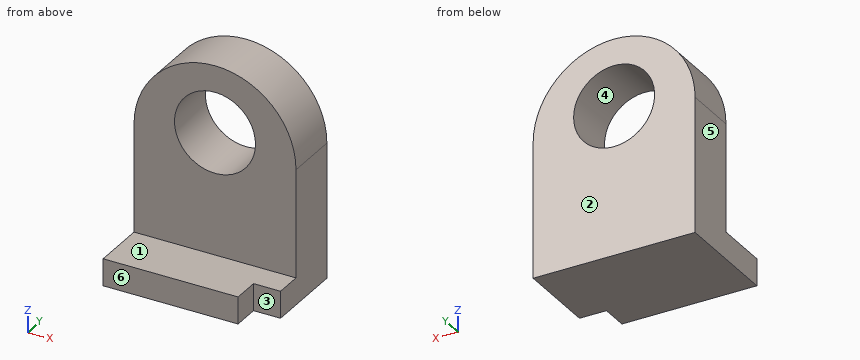
from build123d import *

# Parameters (mm, degrees)
F0_W     = 76.2
F0_H     = 50.8
F1_DEPTH = 12.7
F2_W     = 12.7
F2_H     = 12.7
F3_DEPTH = 12.7
F5_DEPTH = 25.4
F6_R     = 19.05
F7_DEPTH = 25.4


with BuildPart() as f1:
    # F0 (on Top) → F1 (new body)
    with BuildSketch(Plane.XY):
        Rectangle(F0_W, F0_H)
    extrude(amount=F1_DEPTH)

    # F2 (on face) → F3 (cut)
    with BuildSketch(Plane.XY.offset(12.7)):
        with Locations((31.75, -19.05)):
            Rectangle(F2_W, F2_H)
    extrude(amount=-F3_DEPTH, mode=Mode.SUBTRACT)

    # F4 (on Front) → F5 (join)
    with BuildSketch(Plane.XZ):
        with BuildLine():
            Line((-38.1, 12.7), (38.1, 12.7))
            Line((38.1, 12.7), (38.1, 63.5))
            ThreePointArc((38.1, 63.5), (0, 25.4), (-38.1, 63.5))
            Line((-38.1, 63.5), (-38.1, 12.7))
        make_face()
        with BuildLine():
            ThreePointArc((-38.1, 63.5), (0, 25.4), (38.1, 63.5))
            Line((38.1, 63.5), (-38.1, 63.5))
        make_face()
        with BuildLine():
            Line((-38.1, 63.5), (38.1, 63.5))
            ThreePointArc((38.1, 63.5), (0, 101.6), (-38.1, 63.5))
        make_face()
    extrude(amount=-F5_DEPTH)

    # F6 (on face) → F7 (cut)
    with BuildSketch(Plane.XZ):
        with Locations((0, 70.110589)):
            Circle(F6_R)
    extrude(amount=-F7_DEPTH, mode=Mode.SUBTRACT)


solid = f1.part
Can you work these out from the model? Positions are in its coordinate system, mm. Face numbers are marked on the shaded views. A direction names the side the tool comes from. Round coordinates to 2 decimals unless told otherwise and drop trailing zeros. Loops run counter-clockwise (first coordinate to the right, second up) from the corner with the lowest first, then second, coordinate; pieces in that order, holes last. Notation, with made-up numbers: (59, 53.25) - (94, 53.25) arc R14 cw to (94, 71.25) - close; hole circle Ø7 at (63.5, -34.5). An arc over 180 degrees is marked (long way). Write item = value, one per line. Start each with the question number.
(1) If we mould it in two halves opening along X, with no side actions, what happens to the marked faces 4, 5 and 6? For each: released by +X, released by -X, zero draft, split by the parting line, or undercut.
(2) If I drill on probe 1 along Z at (x, y) = (0, 18.75); probe 2 along Y at (x, z) = (5.5, 43.5); probe 3 along Z at (x, y) = (-6, 13), over which ranges is the centre line in solid material (lowest first)? Write a range as [from, to].
(3) For the marked faces 1, 2 and 3, which set-ups out of +Z, -Z, +X, -X, +Y, -Y let a thin tool reach every point of the face, with its end or its side?
(4) For P1, Ø7.5, axis at x = -1, y = -17, coming from the +Z side; P2, Ø14, axis at x = 33, z = 9, coming from the -Y side; P3, Ø3, axis at x = -3.5, z = 45, coming from the -Y side; P4, Ø12, axis at y = -2.5, z = 63.5, coming from the -X side, each with a flat end and sliding along its axis, tell me the tip position at first contact or that it passes through.
(5) If we section it at A-A (x = 0): Please give me the cut outline in (y, z), and give its area (3 significant figures).
(6) If we section it at C-C (x = 13): Please give me the cut outline in (y, z), and give its area (3 significant figures).
(7) If we section it at B-B (z = 88): Please give me the cut outline in (x, y).
(8) If we section it at D-D (y = -17): Please give me the cut outline in (x, z).
Ans:
q1.face_4 = undercut
q1.face_5 = released by -X
q1.face_6 = zero draft
q2.probe_1 = [0, 51.06], [89.16, 101.6]
q2.probe_2 = [0, 25.4]
q2.probe_3 = [0, 52.03], [88.19, 101.12]
q3.face_1 = +Z, +X, -X, -Y
q3.face_2 = +Z, -Z, +X, -X, +Y
q3.face_3 = +Z, -Z, +X, -Y
q4.P1 = 12.7
q4.P2 = -12.7
q4.P3 = 0
q4.P4 = -38.1
q5.outline = (-25.4, 0) - (25.4, 0) - (25.4, 51.06) - (0, 51.06) - (0, 12.7) - (-25.4, 12.7) - close; (0, 89.16) - (25.4, 89.16) - (25.4, 101.6) - (0, 101.6) - close
q5.area = 1,940 mm²
q6.outline = (-25.4, 0) - (25.4, 0) - (25.4, 56.19) - (0, 56.19) - (0, 12.7) - (-25.4, 12.7) - close; (0, 84.04) - (25.4, 84.04) - (25.4, 99.31) - (0, 99.31) - close
q6.area = 2,140 mm²
q7.outline = (-29.18, 0) - (-6.55, 0) - (-6.55, 25.4) - (-29.18, 25.4) - close; (6.55, 0) - (29.18, 0) - (29.18, 25.4) - (6.55, 25.4) - close
q8.outline = (-38.1, 0) - (25.4, 0) - (25.4, 12.7) - (-38.1, 12.7) - close
